CAD build for the part. Positions are in the model's coordinates, mm. A direction names the side the tool comes from. Round coordinates to 2 decimals unless told otherwise and drop trailing zeros. Write each loop counter-clockwise with the first axis right and the second up, starting at its lowest first coordinate (ties: lowest second). Pieces come first, ordered by that corner, then holes. Notation, with made-up numbers: (53.5, -33) -> (112.5, -33) arc R20 cw to (112.5, -13) -> close; hole circle Ø6 at (22, -9.5). An arc over 180 degrees is marked (long way). Put each result on its own line as item: value. Start each with the question number.
1. Saw through at B-B on y = 23.5. List the corners of the cut face in (x, z), and give its area (3 significant figures).
2. Drill centre lines: line 1 (X direction, y = 8.5, z = -2.5); line 2 (X direction, y = 27, z = -7.5); line 3 (Z direction, x = 7, y = 42.5). Where is each one in solid material? Low to high. Write a range as from..to.
3. Saw through at A-A on y = 46. List the corners of the cut face in (x, z), and give its area (3 significant figures).
4. Flat gauge pins, fed straight in: P1, Ø1.5, axis at y = 20, z = -7, coming from the -X side; P2, Ø6, axis at y = 26, z = -4, coming from the +X side. Where does each tip first touch, or does it go through?
5. 3-axis set-ups, long thin cutter, end or side, ignore diameter. For faces 4 (the flat face through (10, 28, 0)), 5 (the flat face through (0, 25, -8.3)), 6 (the cylindrical face through (0, 10, -11)): which of +Z, -Z, +X, -X, +Y, -Y reach the whole face in a straight line?
6. Pull direction X, two halves, no side cores. Call faces 1 (the flat face through (1, 0, -9)), 2 (the cylindrical face through (0.209, 37.325, -9.498)), 3 (the cylindrical face through (-0.275, 38.522, -12.497)): pulls with the +X half, pulls with the -X half, needs draft (parallel to the pull), parting line crosses it, or undercut.
from build123d import *

# Parameters (mm, degrees)
SKETCH_1_R          = 11
SKETCH_1_R_2        = 8
EXTRUDE_1_DEPTH     = 25
SKETCH_2_R          = 12.5
SKETCH_2_R_2        = 9.5
EXTRUDE_2_DEPTH     = 30
CHAMFER_2_SIZE      = 4
FILLET_1_SIZE       = 0.5
FILLET_1_SIZE_2     = 5
FILLET_2_SIZE       = 0.5
FILLET_2_SIZE_2     = 5
SKETCH_3_W          = 25
SKETCH_3_H          = 12.5
CUT_EXTRUDE_2_DEPTH = 58.771100137


with BuildPart() as part:
    # 草图1 → 凸台-拉伸1 (new body)
    with BuildSketch(Plane(origin=(0, 0, 0), x_dir=(1, 0, 0), z_dir=(0, 1, 0))):
        with Locations(Location((0, 0, 0), (0, 0, 270))):
            Circle(SKETCH_1_R)
        with Locations(Location((0, 0, 0), (0, 0, 270))):
            Circle(SKETCH_1_R_2, mode=Mode.SUBTRACT)
    extrude(amount=EXTRUDE_1_DEPTH)

    # 草图2 → 凸台-拉伸2 (add)
    with BuildSketch(Plane(origin=(0, 25, 0), x_dir=(1, 0, 0), z_dir=(0, 1, 0))):
        with Locations(Location((0, 0, 0), (0, 0, 270))):
            Circle(SKETCH_2_R)
        with Locations(Location((0, 0, 0), (0, 0, 270))):
            Circle(SKETCH_2_R_2, mode=Mode.SUBTRACT)
    extrude(amount=EXTRUDE_2_DEPTH)

    # 倒角2
    # the kernel refuses this chamfer: 4 mm, written as the material it adds along each edge
    with BuildSketch(Plane(origin=(0, 25, 0), x_dir=(0, 0, 1), z_dir=(-1, 0, 0))) as chamfer_2_piece_1_section:
        Polygon((11, -CHAMFER_2_SIZE), (11 + CHAMFER_2_SIZE, 0), (11, 0), align=None)
    chamfer_2_piece_1 = revolve(axis=Axis((0, 25, 0), (0, 1, 0)), mode=Mode.PRIVATE)
    chamfer_2_piece_1 = chamfer_2_piece_1 & Plane(origin=(0, 21.745250117, 0), x_dir=(0, 0, 1), z_dir=(0, -1, 0)) * Cylinder(12.5, 60, mode=Mode.PRIVATE)
    add(chamfer_2_piece_1)

    # 圆角1
    # an asymmetric fillet: 5, 0.5 mm, written as the material it takes off along each edge
    with BuildSketch(Plane(origin=(0, 0, 0), x_dir=(0, 0, 1), z_dir=(-1, 0, 0))) as fillet_1_piece_1:
        with BuildLine():
            Bezier((8 + FILLET_1_SIZE, 0), (8, 0), (8, FILLET_1_SIZE_2), weights=[1, 0.707106781, 1])
            Line((8, FILLET_1_SIZE_2), (8, 0))
            Line((8, 0), (8 + FILLET_1_SIZE, 0))
        make_face()
    revolve(axis=Axis((0, 0, 0), (0, 1, 0)), mode=Mode.SUBTRACT)

    # 圆角2
    # an asymmetric fillet: 5, 0.5 mm, written as the material it takes off along each edge
    with BuildSketch(Plane(origin=(0, 55, 0), x_dir=(0, 0, 1), z_dir=(-1, 0, 0))) as fillet_2_piece_1:
        with BuildLine():
            Bezier((9.5 + FILLET_2_SIZE, 0), (9.5, 0), (9.5, -FILLET_2_SIZE_2), weights=[1, 0.707106781, 1])
            Line((9.5, -FILLET_2_SIZE_2), (9.5, 0))
            Line((9.5, 0), (9.5 + FILLET_2_SIZE, 0))
        make_face()
    revolve(axis=Axis((0, 55, 0), (0, 1, 0)), mode=Mode.SUBTRACT)

    # 草图3 → 切除-拉伸2 (cut, through all)
    with BuildSketch(Plane(origin=(0, 55, 0), x_dir=(1, 0, 0), z_dir=(0, 1, 0))):
        with Locations((0, -6.25)):
            Rectangle(SKETCH_3_W, SKETCH_3_H)
    extrude(amount=-CUT_EXTRUDE_2_DEPTH, mode=Mode.SUBTRACT)


solid = part.part
Return value:
1. outline: (-12.5, 0) arc R12.5 ccw to (12.5, 0) -> (8, 0) arc R8 cw to (-8, 0) -> close
1. area: 145 mm^2
2. line 1: x = -10.71..-7.6, 7.6..10.71
2. line 2: x = -10..-5.83, 5.83..10
2. line 3: z = -10.36..-6.42
3. outline: (-12.5, 0) arc R12.5 ccw to (12.5, 0) -> (9.5, 0) arc R9.5 cw to (-9.5, 0) -> close
3. area: 104 mm^2
4. P1: stops at x = -9.05
4. P2: stops at x = 12.46
5. face 4: +Z, +X, -X, +Y, -Y
5. face 5: +Z, +Y
5. face 6: -Z, -Y
6. face 1: needs draft
6. face 2: undercut
6. face 3: parting line crosses it
